Verification items for this drawing (mm, ordinates from the low corner). A direction names the side the tool comes from. Round coordinates to 2 decimals unless told otherwise and drop trailing zeros. Loops run counter-clockwise (first coordinate to the right, second up) from the corner with the lowest first, then second, coordinate; pieces in that order, holes last. Notation, with made-up numbers: M 66,26.5 L 120,26.5 A8 ccw 120,40.5 Z; hole C -9,79.5 d9. An arc over 180 degrees is marked long. Answer as CSV lines item,"result".
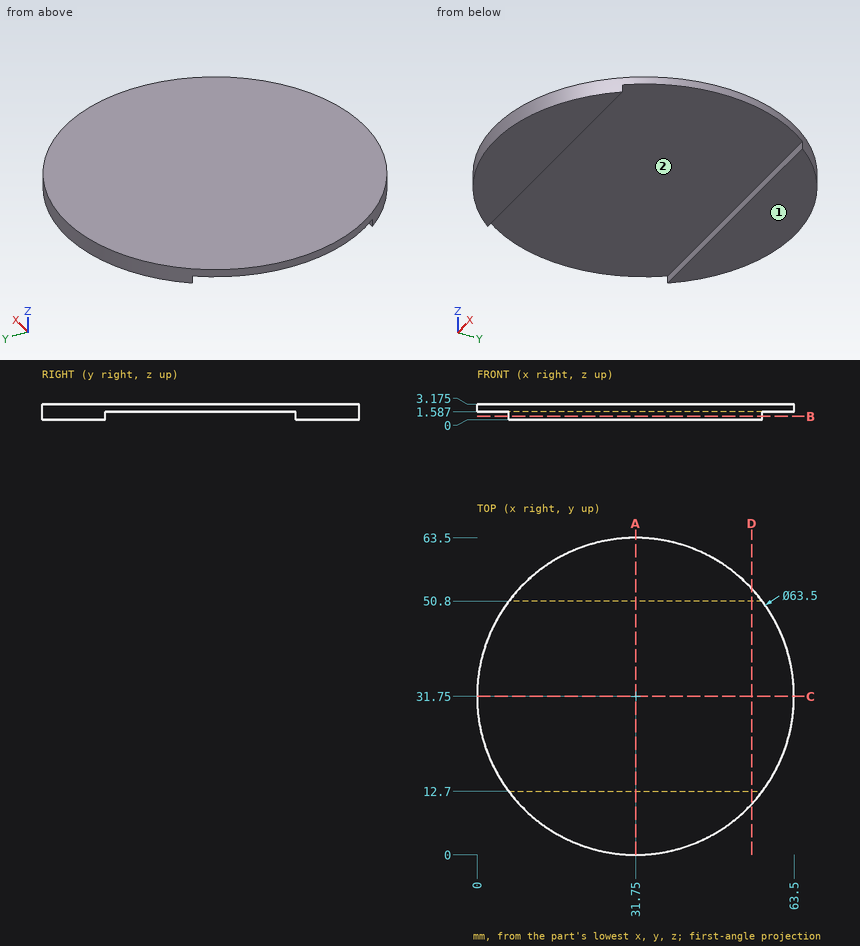
1) Section check D-D (x = 55). Record the cut outline in (y, z) (1 decimal).
Here are the results:
outline,"M 10.1,0 L 12.7,0 L 12.7,1.6 L 50.8,1.6 L 50.8,0 L 53.4,0 L 53.4,3.2 L 10.1,3.2 Z"
2) Section check A-A (x = 31.75). Record the cut outline in (y, z) (1 decimal), plus the area to 3 significant figures.
Here are the results:
outline,"M 0,0 L 12.7,0 L 12.7,1.6 L 50.8,1.6 L 50.8,0 L 63.5,0 L 63.5,3.2 L 0,3.2 Z"
area,"141 mm^2"
3) Section check C-C (y = 31.75). Record the cut outline in (x, z) (1 decimal).
Here are the results:
outline,"M 0,1.6 L 63.5,1.6 L 63.5,3.2 L 0,3.2 Z"
4) Section check B-B (z = 0.7). Record the cut outline in (x, y).
Here are the results:
outline,"M 6.35,12.7 A31.75 ccw 57.15,12.7 Z; M 6.35,50.8 L 57.15,50.8 A31.75 ccw Z"
5) Set-up check for the marked faces 1 and 2: record each of +Z, -Z, +X, -X, +Y, -Y from which the full face is reachable in a straight line by a thin tool's end or side.
Here are the results:
face 1,"-Z, +X, -X, +Y, -Y"
face 2,"-Z, +X, -X"
6) Go/stop test with flat-tipped pins: pin 1 (12 mm diameter, centred on x = 7.5, y = 14.5, fed in from -Z); pin 2 (1.5 mm diameter, centred on x = 51.5, z = 2, fed in from +Y); pin 3 (0.8 mm diameter, centred on x = 41.5, z = 1, fed in from +Y); pin 4 (1.7 mm diameter, centred on x = 27.5, z = 0.5, fed in from -Y). Record where each tip stops, or that it passes through.
Here are the results:
pin 1,"stops at z = 0"
pin 2,"stops at y = 57.19"
pin 3,"stops at y = 62.09"
pin 4,"stops at y = 0.18"
7) Material ranges on probe 1 along Z at (x, y) = (50.5, 29) (1 decimal); probe 2 along Y at (x, z) = (18, 0.35); probe 3 along X at (y, z) = (54.5, 1.15) (1 decimal), recorded low to high.
Here are the results:
probe 1,"z = 1.6 to 3.2"
probe 2,"y = 3.13 to 12.7, 50.8 to 60.37"
probe 3,"x = 9.6 to 53.9"
